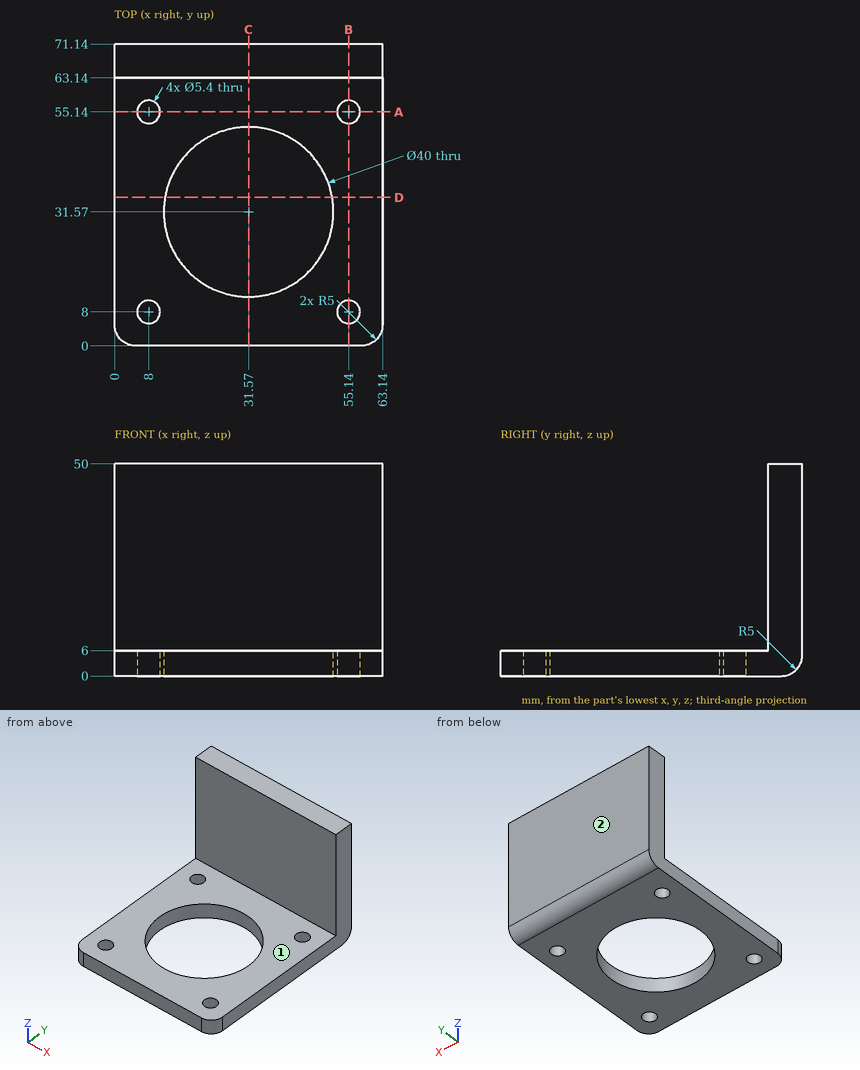
Verification items for this drawing (mm, ordinates from the low corner). A direction names the side the tool comes from. Give positions to 0.01 mm unless a question says otherwise; leave off trailing zeros. Loops run counter-clockwise (first coordinate to the right, second up) from the corner with the lowest first, then second, coordinate; pieces in that order, holes last. Notation, with made-up numbers: (-26.5, 54) - (-20.5, 54) arc R26 cw to (-20.5, 80) - close; hole circle Ø11 at (13.5, -17.75). An arc over 180 degrees is marked (long way). Write item = value, one per line. Start each with the question number.
Q1. Cross-section at D-D, the plane y = 35. Enter the section's corners in (x, z), and give its area (3 significant figures).
Q2. Tool access check on the marked faces 1 and 2. Record the directions out of +Z, -Z, +X, -X, +Y, -Y that give a thin tool (end or side, any length) a straight path to the whole face; none if there is none.
Q3. Depth check by flat-ended pin: P1, Ø13, axis at x = 42.5, z = 36, coming from the -Y side; P2, Ø7, axis at x = 55.14, y = 55.14, coming from the -Z side; P3, Ø8.5, axis at x = 55.14, y = 8, coming from the +Z side. Enter the tip coordinate at first touch or a pass-through.
Q4. Cross-section at C-C, the plane x = 31.57. Enter the section's corners in (y, z).
Q5. Cross-section at B-B, the plane x = 55.14. Enter the section's corners in (y, z).
Q6. Thickness scan on line 1 (Y direction, x = 8, z = 2.6); line 2 (Y direction, x = 8, z = 3); line 3 (Y direction, x = 7, z = 21.5). Record the ranges inside material, lowest first.
Q7. Cross-section at A-A, the plane y = 55.14. Enter the section's corners in (x, z).
Answer key:
q1.outline = (0, 0) - (11.87, 0) - (11.87, 6) - (0, 6) - close; (51.27, 0) - (63.14, 0) - (63.14, 6) - (51.27, 6) - close
q1.area = 142 mm^2
q2.face_1 = +Z, +X, -X, -Y
q2.face_2 = +Z, -Z, +X, -X, +Y
q3.P1 = 63.14
q3.P2 = 0
q3.P3 = 6
q4.outline = (0, 0) - (11.57, 0) - (11.57, 6) - (0, 6) - close; (51.57, 0) - (66.14, 0) arc R5 ccw to (71.14, 5) - (71.14, 50) - (63.14, 50) - (63.14, 6) - (51.57, 6) - close
q5.outline = (0, 0) - (5.3, 0) - (5.3, 6) - (0, 6) - close; (10.7, 0) - (52.44, 0) - (52.44, 6) - (10.7, 6) - close; (57.84, 0) - (66.14, 0) arc R5 ccw to (71.14, 5) - (71.14, 50) - (63.14, 50) - (63.14, 6) - (57.84, 6) - close
q6.line_1 = 0 to 5.3, 10.7 to 52.44, 57.84 to 70.53
q6.line_2 = 0 to 5.3, 10.7 to 52.44, 57.84 to 70.72
q6.line_3 = 63.14 to 71.14
q7.outline = (0, 0) - (5.3, 0) - (5.3, 6) - (0, 6) - close; (10.7, 0) - (52.44, 0) - (52.44, 6) - (10.7, 6) - close; (57.84, 0) - (63.14, 0) - (63.14, 6) - (57.84, 6) - close
